Here's how the part is built. I have some questions about the finished solid (model axes, mm). A direction names the side the tool comes from. Give positions to 0.01 mm unless a question says otherwise; leave off trailing zeros. Write each loop counter-clockwise with the first axis right and the second up, starting at its lowest first coordinate (ties: lowest second). Pieces come first, ordered by that corner, then holes. Notation, with made-up numbers: M -20.5,-25 L 17.5,-25 A28 ccw 17.5,3 Z; hole C -11.75,66 d10. An arc over 180 degrees is marked long. Answer as CSV lines item,"result". Start each with the question number.
Q1. Suppose I cut it at B-B (y = 4). Write out the boundary of the cut face in (x, z), then the cut area to 3 significant figures.
Q2. Thinking about a two-plate mould opening in Z: for faces 3 (the flat face through (4, 0, 3)), 4 (the flat face through (-3.276, 18.444, 3.624)), which applies, +Z half, -Z half, draft (parallel to the pull), parting line (faces both ways), or undercut?
Q3. Suppose I cut it at A-A (x = 0). Count the separate pieces of the cut face and the enclosed holes in it, then the cut area to 3 significant figures.
Q4. For pin 1 (0.7 mm diameter, centred on y = 19, z = -4.5, fed in from -X); pin 2 (3 mm diameter, centred on x = -19, z = 18.5, fed in from +Y); pin 3 (4 mm diameter, centred on x = 12.5, y = 17, fed in from +Z); pin 4 (5 mm diameter, centred on y = 4, z = 10, fed in from -X), each with a flat end and sliding along its axis, tell me the tip position at first contact or that it passes through.
Q5. On a 3-axis mill with a long thin cutter (end or side, diameter ignored), from which of +Z, -Z, +X, -X, +Y, -Y can I reach the whole of each face in a straight line? I mean faces 1 (the flat face through (4.776, 18.444, 1.026)), 2 (the cylindrical face through (-1.141, 10.199, 3.625)). Say none if no direction works.
Q6. If I drill on line 1 along Y through (x, z) = (-4.5, -2.5); line 2 along X through (y, z) = (12, 0); line 3 along X through (y, z) = (11, 0), over which ranges is the centre line in solid material (lowest first)?
```python
from build123d import *

# Parameters (mm, degrees)
SKETCH3_W          = 3
SKETCH3_H          = 8
CUT_EXTRUDE1_DEPTH = 10
CIRPATTERN1_COUNT  = 6
CHAMFER1_SIZE      = 0.5


with BuildPart() as part:
    # Sketch1 → Revolve1 (revolve)
    with BuildSketch(Plane.XY, mode=Mode.PRIVATE) as revolve1_sk:
        with BuildLine():
            Line((0, 30), (10, 30))
            ThreePointArc((10, 30), (24.142135624, 24.142135624), (30, 10))
            ThreePointArc((30, 10), (28.5, 8.5), (27, 10))
            ThreePointArc((27, 10), (22.511577448, 21.509145484), (11.416420028, 26.940890009))
            ThreePointArc((11.416420028, 26.940890009), (7.630166884, 25.6522431), (6, 22))
            Line((6, 22), (6, 0))
            Line((6, 0), (3.8, 0))
            Line((3.8, 0), (3.8, 25))
            Line((3.8, 25), (0, 25))
            Line((0, 25), (0, 30))
        make_face()
    revolve(revolve1_sk.sketch.rotate(Axis((0, 33.38672529, 0), (0, -1, 0)), 90), axis=Axis((0, 33.38672529, 0), (0, -1, 0)))

    # Sketch3 → Cut-Extrude1 (cut)
    with BuildSketch(Plane.XY):
        with Locations((0, 18.5)):
            Rectangle(SKETCH3_W, SKETCH3_H)
    cut_extrude1 = extrude(amount=-CUT_EXTRUDE1_DEPTH, mode=Mode.SUBTRACT)

    # CirPattern1: Cut-Extrude1 ×6 about axis
    cirpattern1_axis = Axis((0, 0, 0), (0, 1, 0))
    for i in range(1, CIRPATTERN1_COUNT):
        add(cut_extrude1.rotate(cirpattern1_axis, i * 360 / CIRPATTERN1_COUNT), mode=Mode.SUBTRACT)

    # Chamfer1
    chamfer1_edges = [part.edges().sort_by_distance(p)[0] for p in [
        (0, 0, -3.8),
    ]]
    chamfer(chamfer1_edges, length=CHAMFER1_SIZE)


solid = part.part
```
Resolved:
1,outline,"C 0,0 d12; hole C 0,0 d7.6"
1,area,"67.7 mm^2"
2,face 3,"draft"
2,face 4,"undercut"
3,separate pieces,"3"
3,enclosed holes,"0"
3,area,"351 mm^2"
4,pin 1,"x = -27.68"
4,pin 2,"y = 23.21"
4,pin 3,"z = 27.03"
4,pin 4,"through"
5,face 1,"none"
5,face 2,"-Y"
6,line 1,"0 to 14.5, 22.5 to 30"
6,line 2,"-29.9 to -26.88, -6 to -3.8, 3.8 to 6, 26.88 to 29.9"
6,line 3,"-29.97 to -26.97, -6 to -3.8, 3.8 to 6, 26.97 to 29.97"
